Input: dimensioned drawing with shaded views. Units: mm. Origin: part minimum x, y, z. A direction names the side the tool comes from. Round coordinates to 2 decimals unless told otherwise and drop trailing zeros. Loops run counter-clockwise (first coordinate to the right, second up) from the corner with the lowest first, then second, coordinate; pieces in that order, holes last. Notation, with made-up numbers: M 10,-17.5 L 58,-17.5 A26 cw 58,15.5 Z; hole C 73.5,-1 d8. An arc over 180 degrees is marked long. Put each result on its own line as item: value. Start each with the question number.
1) Section B-B on z = 25.5. Output: boundary loops of the cut face in (x, y), plus the area to 4 significant figures.
2) Section A-A on y = 9. Output: boundary loops of the cut face in (x, z), plus the area to 3 significant figures.
3) Draft query along X for the marked faces 1, 2 and 3. Return one class per face: +X half, -X half, draft (parallel to the pull), parting line (faces both ways), or undercut.
4) Section D-D on y = 29.5. Output: boundary loops of the cut face in (x, z).
5) Section C-C on x = 16.75. Output: boundary loops of the cut face in (y, z).
6) Line query: probe 1 along X at (y, z) = (11, 27); probe 2 along Z at (x, y) = (15.5, 34); probe 3 along X at (y, z) = (41, 2). Output: solid intervals per line, ascending.
7) Pin query (flat end, axial travel): pin 1 (1.5 mm diameter, centred on y = 40.5, z = 19.5, fed in from -X); pin 2 (4 mm diameter, centred on x = 3, z = 25, fed in from +Y); pin 3 (2.5 mm diameter, centred on x = 10, z = 12.5, fed in from +Y). Return the tip coordinate at first contact, or that it passes through.
8) Reachability of the marked faces 4, 5 and 6 from +Z, -Z, +X, -X, +Y, -Y: full face, straight path, thin tool, end or side. Return the list, or none.
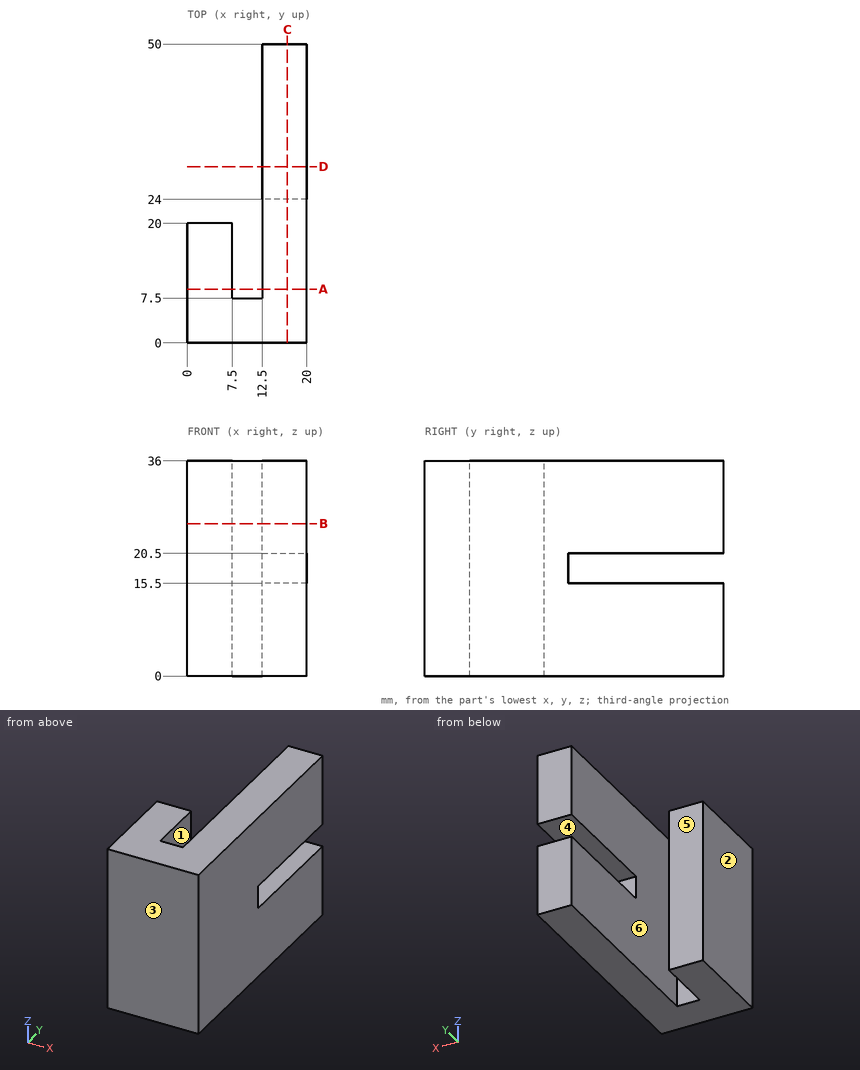
Geometry results:
1. outline: M 0,0 L 20,0 L 20,50 L 12.5,50 L 12.5,7.5 L 7.5,7.5 L 7.5,20 L 0,20 Z
1. area: 562.5 mm²
2. outline: M 0,0 L 7.5,0 L 7.5,36 L 0,36 Z; M 12.5,0 L 20,0 L 20,36 L 12.5,36 Z
2. area: 540 mm²
3. face 1: undercut
3. face 2: -X half
3. face 3: draft
4. outline: M 12.5,0 L 20,0 L 20,15.5 L 12.5,15.5 Z; M 12.5,20.5 L 20,20.5 L 20,36 L 12.5,36 Z
5. outline: M 0,0 L 50,0 L 50,15.5 L 24,15.5 L 24,20.5 L 50,20.5 L 50,36 L 0,36 Z
6. probe 1: x = 0 to 7.5, 12.5 to 20
6. probe 2: z = 0 to 15.5, 20.5 to 36
6. probe 3: x = 12.5 to 20
7. pin 1: passes through
7. pin 2: stops at y = 20
7. pin 3: stops at y = 7.5
8. face 4: +X, -X, +Y
8. face 5: +Z, -Z, -X, +Y
8. face 6: +Z, -Z, +Y
